Can you work these out from the drawing? Everything is in mm from the part's minimum corner. A direction names the side the tool comes from. Coordinates: 2 decimals unless noted, no trailing zeros. Loops run counter-clockwise (first coordinate to the right, second up) from the corner with the lowest first, then second, coordinate; pieces in that order, holes last. Notation, with made-up numbers: M -5,-4.5 L 53,-4.5 A22 ccw 53,20.5 Z; hole C 85,22.25 d8. An arc over 180 degrees is marked long. Use CSV: the item, a comma, the result in double quotes. Start each with the question number.
Q1. Please list where these lines run through material, in increasing order: probe 1 along Z at (x, y) = (15, 8.5); probe 2 along Y at (x, z) = (15.25, 2). Write a range as [from, to].
Q2. If we section it at C-C (z = 17): Please give me the cut outline in (x, y), and give its area (3 significant figures).
Q3. If we mould it in two halves opening along X, with no side actions, what happens to the marked faces 1, 2 and 3? For each: +X half, -X half, draft (parallel to the pull), parting line (faces both ways), or undercut.
Q4. If we section it at B-B (x = 13.15): Please give me the cut outline in (y, z), and give its area (3 significant figures).
Q5. If we section it at D-D (y = 7.5): Please give me the cut outline in (x, z), and give its area (3 significant figures).
Q6. For pin 1 Ø8 at (x, z) = (8, 17.5) entering from +Y; pin 2 Ø3 at (x, y) = (20.5, 16) entering from +Z; pin 3 Ø1.8 at (x, z) = (21.65, 19.85) entering from -Y, each with a flat end and sliding along its axis, tell me the tip position at first contact or that it passes through.
Q7. If we section it at A-A (y = 18): Please give me the cut outline in (x, z).
Q8. Which directions (+Z, -Z, +X, -X, +Y, -Y) give clear straight access to the entire face, cutting with the end or side of a thin tool? Please do the marked faces 4 and 5.
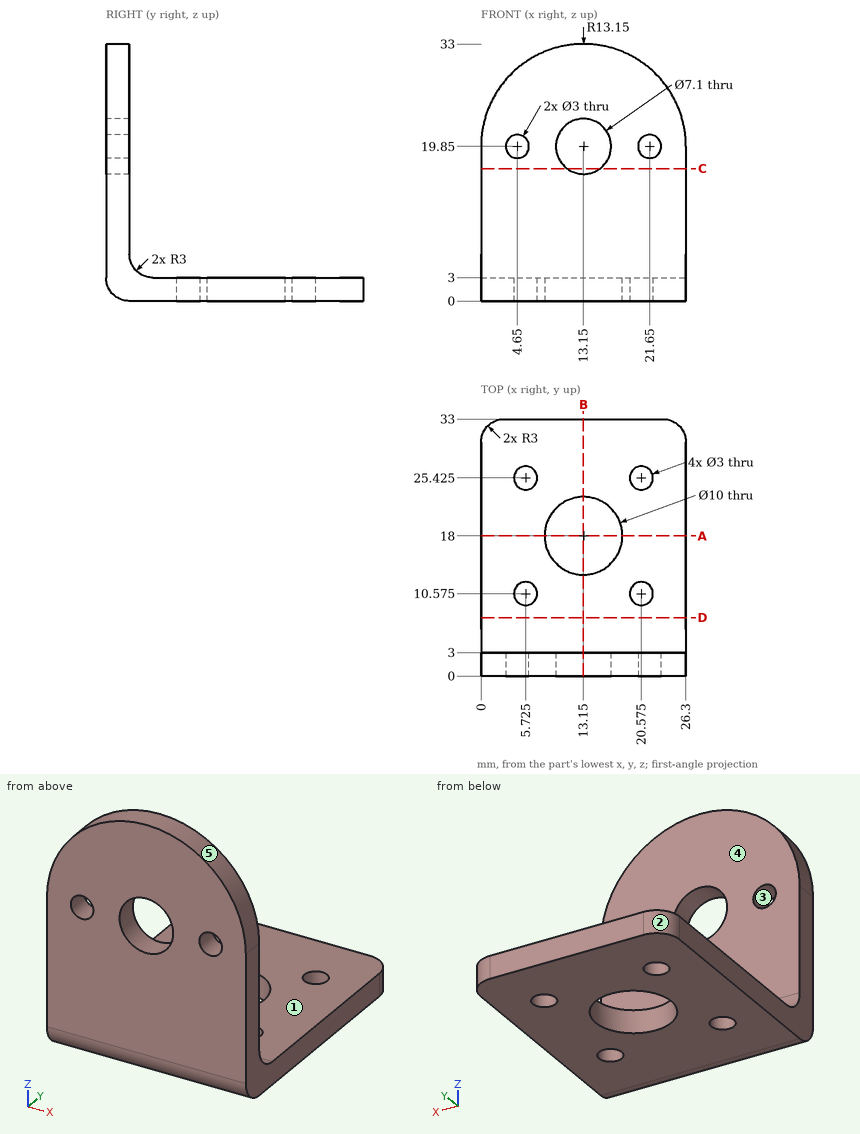
Results below:
1,probe 1,"[0, 3]"
1,probe 2,"[0.17, 13.46], [22.54, 33]"
2,outline,"M 0,0 L 11.03,0 L 11.03,3 L 0,3 Z; M 15.27,0 L 26.3,0 L 26.3,3 L 15.27,3 Z"
2,area,"66.2 mm^2"
3,face 1,"draft"
3,face 2,"-X half"
3,face 3,"undercut"
4,outline,"M 0,3 A3 ccw 3,0 L 13,0 L 13,3 L 6,3 A3 cw 3,6 L 3,16.3 L 0,16.3 Z; M 0,23.4 L 3,23.4 L 3,33 L 0,33 Z; M 23,0 L 33,0 L 33,3 L 23,3 Z"
4,area,"138 mm^2"
5,outline,"M 0,0 L 26.3,0 L 26.3,3 L 0,3 Z"
5,area,"78.9 mm^2"
6,pin 1,"y = 3"
6,pin 2,"z = 3"
6,pin 3,"through"
7,outline,"M 0,0 L 8.15,0 L 8.15,3 L 0,3 Z; M 18.15,0 L 26.3,0 L 26.3,3 L 18.15,3 Z"
8,face 4,"+Z, +X, -X, +Y"
8,face 5,"+Z, +Y, -Y"
